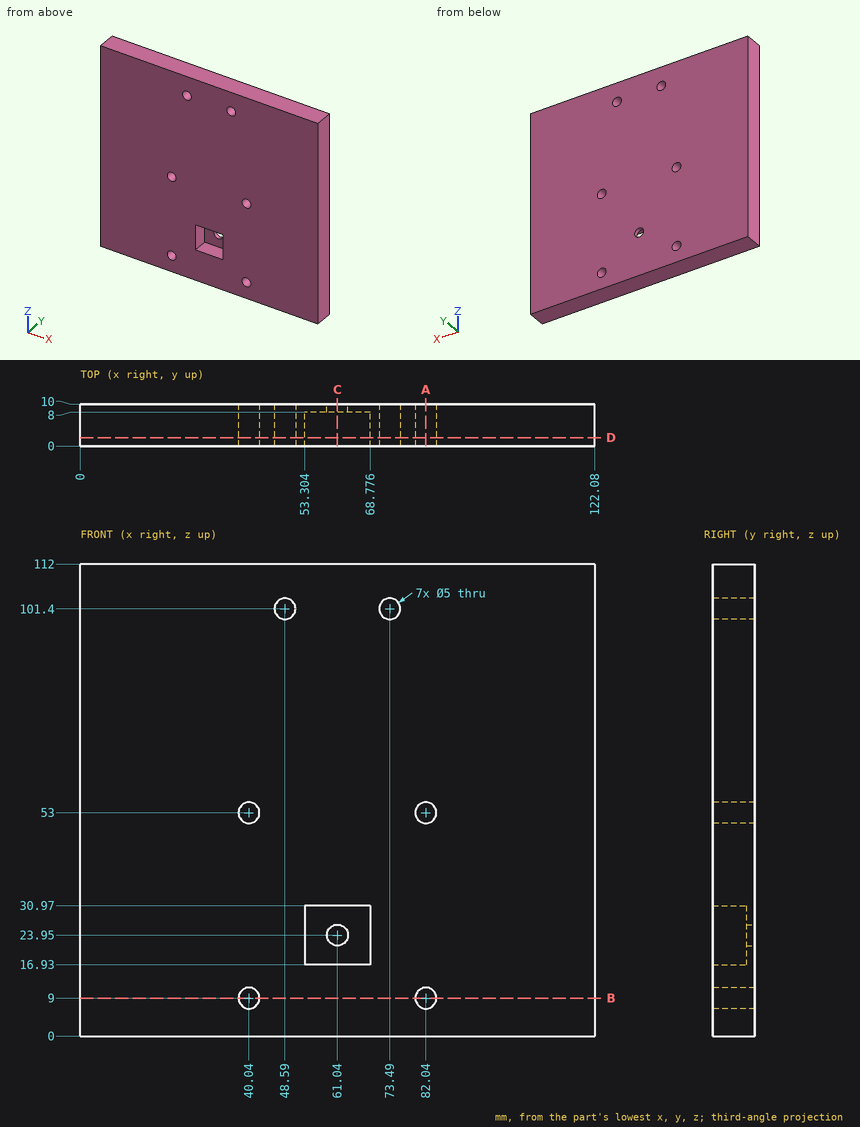
Design review of the part shown in the three views and the two pictorial views. Dimensions are in mm from the part's minimum x, y and z. Round coordinates to 2 decimals unless told otherwise and drop trailing zeros. Loops run counter-clockwise (first coordinate to the right, second up) from the corner with the lowest first, then second, coordinate; pieces in that order, holes last. Notation, with made-up numbers: (45.25, -6) - (85.25, -6) arc R17 cw to (85.25, 14) - close; hole circle Ø5 at (6.25, 7.25). An arc over 180 degrees is marked (long way). Use CSV: the item, a comma, the result in double quotes.
(1) Take a section at A-A, the plane x = 82.04. Give the boundary of the cut face in (y, z), plus the area to 3 significant figures.
Working result:
outline,"(0, 0) - (10, 0) - (10, 6.5) - (0, 6.5) - close; (0, 11.5) - (10, 11.5) - (10, 50.5) - (0, 50.5) - close; (0, 55.5) - (10, 55.5) - (10, 112) - (0, 112) - close"
area,"1,020 mm^2"
(2) For line 1 (Z direction, x = 82.04, y = 6.25); line 2 (X direction, y = 4.5, z = 9); line 3 (X direction, y = 6, z = 30.5), list the stretches that pass through material, from the lowest coordinate up.
Working result:
line 1,"z = 0 to 6.5, 11.5 to 50.5, 55.5 to 112"
line 2,"x = 0 to 37.54, 42.54 to 79.54, 84.54 to 122.08"
line 3,"x = 0 to 53.3, 68.78 to 122.08"
(3) Clearance check with a flat-ended pin moving along its axis: P1, Ø4, axis at x = 40.04, z = 53, coming from the -Y side. State where the tip first meets the part, or that it passes through.
Working result:
P1,"passes through"
(4) Take a section at C-C, the plane x = 61.04. Give the boundary of the cut face in (y, z).
Working result:
outline,"(0, 0) - (10, 0) - (10, 21.45) - (8, 21.45) - (8, 16.93) - (0, 16.93) - close; (0, 30.97) - (8, 30.97) - (8, 26.45) - (10, 26.45) - (10, 112) - (0, 112) - close"
(5) Take a section at D-D, the plane y = 2. Give the boundary of the cut face in (x, z).
Working result:
outline,"(0, 0) - (122.08, 0) - (122.08, 112) - (0, 112) - close; hole circle Ø5 at (40.04, 9); hole circle Ø5 at (40.04, 53); hole circle Ø5 at (48.59, 101.4); hole (53.3, 16.93) - (68.78, 16.93) - (68.78, 30.97) - (53.3, 30.97) - close; hole circle Ø5 at (73.49, 101.4); hole circle Ø5 at (82.04, 9); hole circle Ø5 at (82.04, 53)"
(6) Take a section at B-B, the plane z = 9. Give the boundary of the cut face in (x, y).
Working result:
outline,"(0, 0) - (37.54, 0) - (37.54, 10) - (0, 10) - close; (42.54, 0) - (79.54, 0) - (79.54, 10) - (42.54, 10) - close; (84.54, 0) - (122.08, 0) - (122.08, 10) - (84.54, 10) - close"
